Drawing for the job (mm, zero at the part's lowest x, y, z). Coordinates: 2 decimals unless noted, no trailing zeros. Order: outer loops, then holes, each group sorted by start corner. A loop starts at its lowest first (then second) coordinate and runs counter-clockwise, first axis right, second up. Notation, with made-up numbers: (-27, 24) - (-4, 24) arc R33 ccw to (-4, 56) - close; hole circle Ø3 at (22.5, -6.75). An arc over 180 degrees is marked (long way). Answer as CSV lines item,"result". Start each with the question number.
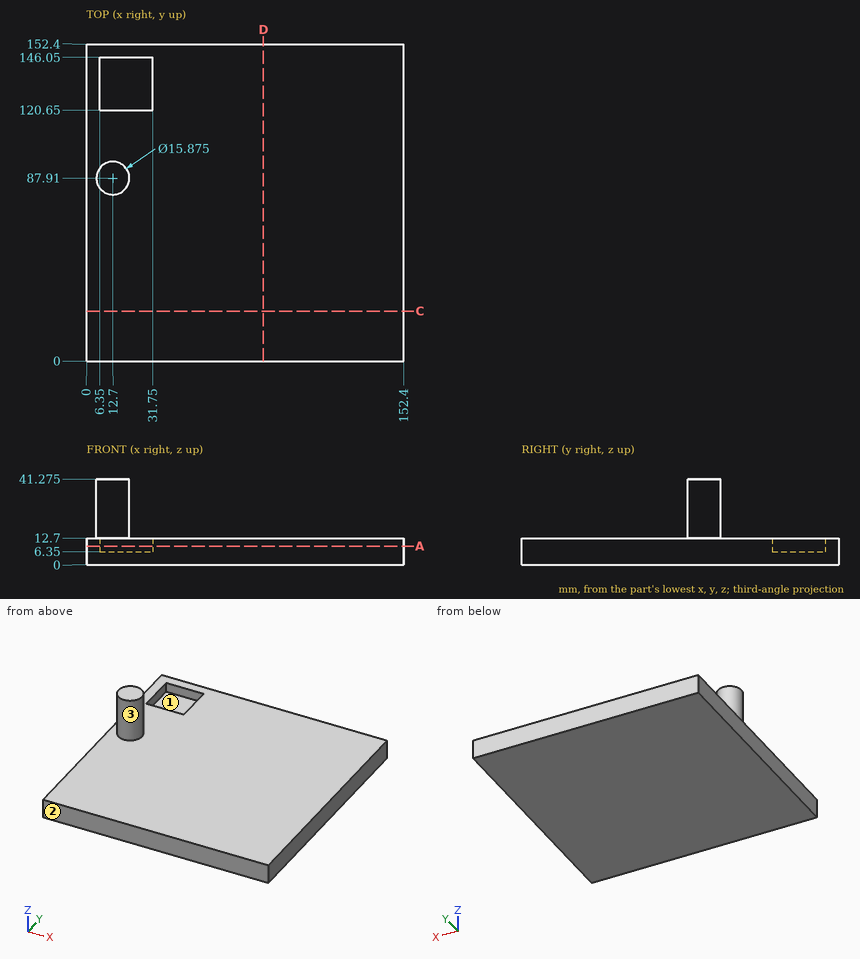
(1) Band-saw the part on C-C on y = 24. List the corners of the cut face in (x, z).
(2) Probe L1, parallel to Z at x = 71, y = 28; L2, parallel to Z at x = 21, y = 133.5; L3, parallel to Y at x = 18, z = 37. List the from-to ranges inside material, lowest first. Write a range as [from, to].
(3) Drop flat-ended pins along their axis: pin 1 Ø1 at (y, z) = (83, 23.5) entering from -X; pin 2 Ø7.5 at (x, y) = (13.5, 135.5) entering from +Z; pin 3 Ø12 at (x, y) = (36.5, 114) entering from +Z; pin 4 Ø2 at (x, z) = (63.5, 15) entering from -Y. Give the stop position or say it passes through.
(4) Pull direction X, two halves, no side cores. Call the marked faces 1, 2 and 3: +X half, -X half, draft (parallel to the pull), parting line (faces both ways), or undercut.
(5) Band-saw the part on A-A on z = 9. List the corners of the cut face in (x, y).
Filled in:
1,outline,"(0, 0) - (152.4, 0) - (152.4, 12.7) - (0, 12.7) - close"
2,L1,"z = [0, 12.7]"
2,L2,"z = [0, 6.35]"
2,L3,"y = [82, 93.82]"
3,pin 1,"stops at x = 6.1"
3,pin 2,"stops at z = 6.35"
3,pin 3,"stops at z = 12.7"
3,pin 4,"passes through"
4,face 1,"undercut"
4,face 2,"draft"
4,face 3,"parting line"
5,outline,"(0, 0) - (152.4, 0) - (152.4, 152.4) - (0, 152.4) - close; hole (6.35, 120.65) - (31.75, 120.65) - (31.75, 146.05) - (6.35, 146.05) - close"
